```python
from build123d import *

# Parameters (mm, degrees)
SKETCH1_R               = 3.175
EXTRUDE1_DEPTH          = 2.778125
SKETCH7_OUTSIDE_W       = 104.672
SKETCH7_OUTSIDE_H       = 106.392
SKETCH7_OUTSIDE_R       = 5.55625
EXTRUDE2_DEPTH          = 25.4
EXTRUDE2_DRAFT          = -60
MIRROR1_COPY_1_SKETCH_W = 104.672
MIRROR1_COPY_1_SKETCH_H = 106.392
MIRROR1_COPY_1_SKETCH_R = 5.55625
MIRROR1_COPY_1_DEPTH    = 25.4
MIRROR1_COPY_1_DRAFT    = -60


with BuildPart() as part:
    # Sketch1 → Extrude1 (new, symmetric)
    with BuildSketch(Plane.XY):
        Polygon((-5.55625, 3.207902433), (-5.55625, -3.207902433), (0, -6.415804866), (5.55625, -3.207902433), (5.55625, 3.207902433), (0, 6.415804866), align=None)
        Circle(SKETCH1_R, mode=Mode.SUBTRACT)
    extrude(amount=EXTRUDE1_DEPTH, both=True)


with BuildPart() as extrude2_tool:
    # Sketch7 outside → Extrude2 (with draft: the straight prism first)
    with BuildSketch(Plane.XY.offset(2.778125)):
        Rectangle(SKETCH7_OUTSIDE_W, SKETCH7_OUTSIDE_H)
        Circle(SKETCH7_OUTSIDE_R, mode=Mode.SUBTRACT)
    extrude(amount=-EXTRUDE2_DEPTH)
    # Extrude2: the draft: its side faces are tilted about the plane it starts from
    extrude2_sides = [extrude2_tool.faces().sort_by_distance(p)[0] for p in [
        (0, -53.196, -9.921875),
        (52.336, 0, -9.921875),
        (0, 53.196, -9.921875),
        (-52.336, 0, -9.921875),
        (-5.55625, 0, -9.921875),
    ]]
    draft(extrude2_sides, Plane.XY.offset(2.778125), EXTRUDE2_DRAFT)


with BuildPart() as part_1:
    add(part.part)

    # Extrude2: cut by extrude2_tool
    add(extrude2_tool.part, mode=Mode.SUBTRACT)


with BuildPart() as mirror1_copy_1_tool:
    # Mirror1 copy 1 sketch → Mirror1 copy 1 (with draft: the straight prism first)
    with BuildSketch(Plane(origin=(0, 0, -2.778125), x_dir=(1, 0, 0), z_dir=(0, 0, -1))):
        Rectangle(MIRROR1_COPY_1_SKETCH_W, MIRROR1_COPY_1_SKETCH_H)
        Circle(MIRROR1_COPY_1_SKETCH_R, mode=Mode.SUBTRACT)
    extrude(amount=-MIRROR1_COPY_1_DEPTH)
    # Mirror1 copy 1: the draft: its side faces are tilted about the plane it starts from
    mirror1_copy_1_sides = [mirror1_copy_1_tool.faces().sort_by_distance(p)[0] for p in [
        (0, -53.196, 9.921875),
        (52.336, 0, 9.921875),
        (0, 53.196, 9.921875),
        (-52.336, 0, 9.921875),
        (-5.55625, 0, 9.921875),
    ]]
    draft(mirror1_copy_1_sides, Plane(origin=(0, 0, -2.778125), x_dir=(1, 0, 0), z_dir=(0, 0, -1)), MIRROR1_COPY_1_DRAFT)


with BuildPart() as part_2:
    add(part_1.part)

    # Mirror1 copy 1: cut by mirror1_copy_1_tool
    add(mirror1_copy_1_tool.part, mode=Mode.SUBTRACT)


solid = part_2.part
```
Geometry: final body of the model. Coordinates: model frame, mm. Round coordinates to 2 decimals unless told otherwise and drop trailing zeros. Write each loop counter-clockwise with the first axis right and the second up, starting at its lowest first coordinate (ties: lowest second). Pieces come first, ordered by that corner, then holes.
Item 1: Mould query, pull axis X, two halves, no side actions, for faces 1 (the face through (-0.69, -3.1, -0.04)), 2 (the face through (4.996, -2.868, -2.66)), 3 (the face through (-4.98, -2.89, -2.66)), 4 (the face through (0.01, -5.76, -2.66)). Classes: +X half, -X half, draft (parallel to the pull), parting line (faces both ways), or undercut.
Item 2: Section query A-A (z = 1.55). Return loops of the section in (x, y) (3 decimals), plus the area to 3 significant figures.
Item 3: Material intervals for L1, parallel to Y at x = -1.5, z = 1.6; L2, parallel to Y at x = 0.25, z = 1.7; L3, parallel to X at y = -1.25, z = 0.15, sorted ascending.
Item 4: Pin query (flat end, axial travel): P1, Ø1.5, axis at x = -3.5, z = -2, coming from the -Y side; P2, Ø1.5, axis at x = -3, z = 2, coming from the -Y side. Return the tip coordinate at first contact, or that it passes through.
Completed:
1. face 1: undercut
1. face 2: +X half
1. face 3: -X half
1. face 4: parting line
2. outline: (-5.556, -3.208) - (0, -6.416) - (5.556, -3.208) - (5.556, 3.208) - (0, 6.416) - (-5.556, 3.208) - close; hole circle Ø6.35 at (0, 0)
2. area: 75.3 mm2
3. L1: y = -5.55 to -2.8, 2.8 to 5.55
3. L2: y = -6.27 to -3.17, 3.17 to 6.27
3. L3: x = -5.56 to -2.92, 2.92 to 5.56
4. P1: stops at y = -4.83
4. P2: stops at y = -5.12
